```python
from build123d import *

# Parameters (mm, degrees)
BOSS_EXTRUDE1_DEPTH = 10
SKETCH2_R           = 30
CUT_EXTRUDE1_DEPTH  = 11


with BuildPart() as part:
    # Sketch1 → Boss-Extrude1 (new body)
    with BuildSketch(Plane(origin=(0, 0, 0), x_dir=(1, 0, 0), z_dir=(0, 1, 0))):
        with BuildLine():
            Line((-53.449605369, 12.68115942), (200.724637681, 12.68115942))
            Line((200.724637681, 12.68115942), (200.724637681, -27.31884058))
            Line((200.724637681, -27.31884058), (-53.449605369, -27.31884058))
            ThreePointArc((-53.449605369, -27.31884058), (-149.275362319, -7.31884058), (-53.449605369, 12.68115942))
        make_face()
    extrude(amount=BOSS_EXTRUDE1_DEPTH)

    # Sketch2 → Cut-Extrude1 (cut, through all)
    with BuildSketch(Plane(origin=(0, 10, 0), x_dir=(1, 0, 0), z_dir=(0, 1, 0))):
        with Locations((-98.874058495, -8.131832766)):
            Circle(SKETCH2_R)
    extrude(amount=-CUT_EXTRUDE1_DEPTH, mode=Mode.SUBTRACT)


solid = part.part
```
Design review of the part built by this model. Coordinates are the model's own, in mm. A direction names the side the tool comes from. Coordinates: 2 decimals unless noted, no trailing zeros. Loops run counter-clockwise (first coordinate to the right, second up) from the corner with the lowest first, then second, coordinate; pieces in that order, holes last. Notation, with made-up numbers: M 49.25,11 L 56.25,11 A32 ccw 56.25,48 Z; hole C 10.5,33.5 d3. An arc over 180 degrees is marked long. One line per question, with ' | ' between items.
(1) Wall thickness on probe 1 along X at (y, z) = (5.75, 6.5); probe 2 along Z at (x, y) = (27, 9.75); probe 3 along X at (y, z) = (6.5, 3.5): over which ranges is each line inside the solid? List them lowest first.
Filled in:
probe 1: x = -149.27 to -128.83, -68.92 to 200.72 | probe 2: z = -12.68 to 27.32 | probe 3: x = -149.13 to -128.51, -69.23 to 200.72
(2) Machinability: for faces 1 (the face through (28, 0, 7)), 2 (the face through (75, 5, 27.319)), 3 (the face through (72, 5, -12.681)), which of the approach directions +Z, -Z, +X, -X, +Y, -Y give a long, thin tool a straight path to every point of the face, cutting with its end or side? Answer none if there is none.
Filled in:
face 1: +Z, -Z, +X, -X, -Y | face 2: +Z, +X, +Y, -Y | face 3: -Z, +X, +Y, -Y
(3) Draft analysis for pull direction X (two halves, no side actions). For faces 4 (the face through (28, 10, 7)), 5 (the face through (-128.845, 5.07, 6.813)), 6 (the face through (200.725, 5, 7)), state which applies: released by +X, released by -X, zero draft, split by the parting line, or undercut.
Filled in:
face 4: zero draft | face 5: undercut | face 6: released by +X
(4) We need section A-A (x = -78). Give the boundary of the cut face in (y, z).
Filled in:
outline: M 0,-37.93 L 10,-37.93 L 10,-13.42 L 0,-13.42 Z; M 0,29.68 L 10,29.68 L 10,52.57 L 0,52.57 Z
(5) We need section B-B (z = 34). Give the boundary of the cut face in (x, y), and give its area (3 significant figures).
Filled in:
outline: M -141.56,0 L -114.07,0 L -114.07,10 L -141.56,10 Z; M -83.68,0 L -56.99,0 L -56.99,10 L -83.68,10 Z | area: 542 mm^2
(6) For pin 1 Ø3 at (x, y) = (24.5, 7) entering from +Z; pin 2 Ø6 at (y, z) = (6.5, -32.5) entering from +X; pin 3 Ø1.5 at (x, y) = (140.5, 8.5) entering from -Z, all flat-tipped, find the tip position at first contact; note any pin that passes through.
Filled in:
pin 1: stops at z = 27.32 | pin 2: stops at x = -65.45 | pin 3: stops at z = -12.68
(7) We need section C-C (y = 1.5). Give the boundary of the cut face in (x, z).
Filled in:
outline: M -53.45,-12.68 L 200.72,-12.68 L 200.72,27.32 L -53.45,27.32 A50 ccw long Z; hole C -98.87,8.13 d60
(8) We need section D-D (x = 4). Give the boundary of the cut face in (y, z).
Filled in:
outline: M 0,-12.68 L 10,-12.68 L 10,27.32 L 0,27.32 Z
